Design review of the part built by this model. Coordinates are the model's own, in mm. A direction names the side the tool comes from. Give positions to 0.01 mm unless a question says otherwise; leave off trailing zeros. Write each loop counter-clockwise with the first axis right and the second up, starting at its lowest first coordinate (ties: lowest second). Pieces come first, ordered by that corner, then holes. Notation, with made-up numbers: M 47,-35 L 56,-35 A15 cw 56,-25 Z; hole C 68.5,5.25 d6. An arc over 180 degrees is marked long. Write each question's results on one line, items separated by ' | '. Start each with the question number.
from build123d import *

# Parameters (mm, degrees)
SKETCH8_R           = 4.445
CUT_EXTRUDE2_DEPTH  = 10.16
CIRPATTERN1_COUNT   = 6
SKETCH10_R          = 40.005
CUT_EXTRUDE4_DEPTH  = 125.434078974
REVOLVE4_ANGLE      = 180
CIRPATTERN2_COUNT   = 4
SKETCH16_R          = 5.079288484
BOSS_EXTRUDE1_DEPTH = 10.16


with BuildPart() as part:
    # Sketch1 → Revolve1 (revolve)
    with BuildSketch(Plane(origin=(0, 0, 0), x_dir=(0, 0, -1), z_dir=(1, 0, 0))):
        Polygon((0, 0), (0, -25.4), (6.35, -25.4), (6.35, -50.8), (12.7, -50.8), (12.7, 0), align=None)
    revolve(axis=Axis((0, 24.668312757, -50.8), (0, -1, 0)))

    # Sketch8 → Cut-Extrude2 (cut, symmetric)
    with BuildSketch(Plane.XY.offset(-6.707819403)):
        with Locations(Location((0, -38.1, 0), (0, 0, 270))):
            Circle(SKETCH8_R)
    cut_extrude2 = extrude(amount=CUT_EXTRUDE2_DEPTH, both=True, mode=Mode.SUBTRACT)

    # CirPattern1: Cut-Extrude2 ×6 about axis
    cirpattern1_axis = Axis((0, 24.668312757, -50.8), (0, 1, 0))
    for i in range(1, CIRPATTERN1_COUNT):
        add(cut_extrude2.rotate(cirpattern1_axis, i * 360 / CIRPATTERN1_COUNT), mode=Mode.SUBTRACT)

    # Sketch10 → Cut-Extrude4 (cut, through all)
    with BuildSketch(Plane.XZ.offset(50.8)):
        with Locations(Location((0, -50.8, 0), (0, 0, 270))):
            Circle(SKETCH10_R)
    extrude(amount=-CUT_EXTRUDE4_DEPTH, mode=Mode.SUBTRACT)

    # Sketch14 → Revolve4 (revolve)
    with BuildSketch(Plane(origin=(0, 0, 0), x_dir=(1, 0, 0), z_dir=(0, 1, 0))):
        with BuildLine():
            Line((7.253808844, 11.458135755), (0.649808844, 10.800277833))
            ThreePointArc((0.649808844, 10.800277833), (3.622879883, 14.431206794), (7.253808844, 11.458135755))
        make_face()
    revolve4 = revolve(axis=Axis((0.649808844, 0, -10.800277833), (-0.9950750421165625, 0, 0.09912447001987663)), revolution_arc=REVOLVE4_ANGLE)

    # CirPattern2: Revolve4 ×4 about axis
    cirpattern2_axis = Axis((0, 0, -50.8), (0, 1, 0))
    for i in range(1, CIRPATTERN2_COUNT):
        add(revolve4.rotate(cirpattern2_axis, i * 360 / CIRPATTERN2_COUNT))

    # Sketch16 → Boss-Extrude1 (add)
    with BuildSketch(Plane(origin=(0, 0, 0), x_dir=(1, 0, 0), z_dir=(0, 1, 0))):
        with Locations(Location((4.452646476, 5.350182374, 0), (0, 0, 270))):
            Circle(SKETCH16_R)
    extrude(amount=BOSS_EXTRUDE1_DEPTH)


solid = part.part
Q1. The part is to be moulded in two halves that separate along X. For faces 1 (the flat face through (45, -25.4, -51)), 2 (the cylindrical face through (1.702, -42.206, -92.938)), 3 (the cylindrical face through (-0.506, 5.009, -6.451)), say which applies: pulls with the +X half, pulls with the -X half, needs draft (parallel to the pull), parting line crosses it, or undercut.
Q2. We need section D-D on y = -29. Write out the cut boundary in (x, z) (3 decimals), and give its area (3 significant figures).
Q3. We need section A-A on y = -38.1. Write out the cut boundary in (x, z) (3 decimals), and give its area (3 significant figures).
Q4. For faces 4 (the flat face through (5, 10.16, -5)), 5 (the cylindrical face through (-13.352, -38.278, -8.403)), list the 3-axis set-ups (+Z, -Z, +X, -X, +Y, -Y) from which the entire face can be reached by the end or side of a thin tool; tool diameter is ignored.
Q5. Wall thickness on line 1 along Y through (x, z) = (0, -8.1) (3 decimals); line 2 along X through (y, z) = (-16, -50); line 3 along X through (y, z) = (-33.5, -50.8) (3 decimals): over which ranges is each line inside the solid? List them lowest first. Write a range as from..to.
Q6. We need section C-C on y = -6.5. Write out the cut boundary in (x, z) (3 decimals).
Q7. We need section B-B on x = -9. Write out the cut boundary in (y, z), and give its area (3 significant figures).
Q8. For pin 1 Ø1.5 at (x, z) = (24.5, -16) entering from +Y; pin 2 Ø8 at (x, y) = (-16, -26.5) entering from +Z; pin 3 Ø10 at (x, y) = (0, -38.1) entering from -Z, all flat-tipped, find the tip position at first contact; note any pin that passes through.
Answer sheet:
1) face 1: needs draft | face 2: undercut | face 3: parting line crosses it
2) outline: C 0,-50.8 d88.9; hole C 0,-50.8 d80.01 | area: 1,180 mm^2
3) outline: M -40.524,-69.064 L -36.653,-66.829 A40.005 cw -36.653,-34.771 L -40.524,-32.536 A44.45 ccw Z; M -36.079,-76.763 A44.45 ccw -4.445,-95.027 L -4.445,-90.557 A40.005 cw -32.208,-74.528 Z; M -36.079,-24.837 L -32.208,-27.072 A40.005 cw -4.445,-11.043 L -4.445,-6.573 A44.45 ccw Z; M 4.445,-95.027 A44.45 ccw 36.079,-76.763 L 32.208,-74.528 A40.005 cw 4.445,-90.557 Z; M 4.445,-11.043 A40.005 cw 32.208,-27.072 L 36.079,-24.837 A44.45 ccw 4.445,-6.573 Z; M 36.653,-66.829 L 40.524,-69.064 A44.45 ccw 40.524,-32.536 L 36.653,-34.771 A40.005 cw Z | area: 942 mm^2
4) face 4: +Z, -Z, +X, -X, +Y | face 5: -Y
5) line 1: -50.8..-42.545, -33.655..0 | line 2: -50.79..-40, 40..50.79 | line 3: -44.45..-40.005, 40.005..44.45
6) outline: C 0,-50.8 d101.6; hole C 0,-50.8 d80.01
7) outline: M -50.8,-94.33 L -25.4,-94.33 L -25.4,-100.8 L 0,-100.8 L 0,-89.78 L -50.8,-89.78 Z; M -50.8,-11.82 L 0,-11.82 L 0,-0.8 L -25.4,-0.8 L -25.4,-7.27 L -50.8,-7.27 Z | area: 791 mm^2
8) pin 1: y = 0 | pin 2: z = -1.48 | pin 3: z = -95.25
